The listing builds one solid part. Answer for the finished solid, in the listing's coordinates (mm). A direction names the side the tool comes from. Give positions to 0.01 mm unless a question says otherwise; leave off trailing zeros. Order: outer loops, then holes, each group sorted by start corner. A loop starts at its lowest first (then second) coordinate and runs counter-clockwise, first axis right, second up. Notation, with made-up numbers: (24, -25) - (75, -25) arc R18 cw to (75, -3) - close; hole circle Ø4 at (-20, 85). An arc over 180 degrees is marked (long way). Write each question's results on one line, items separated by ' | '. Start each with the question number.
1. Flat-ended cylindrical pins translate along their axes: pin 1 (2.5 mm diameter, centred on x = -33.5, z = -31.5, fed in from -Y); pin 2 (5 mm diameter, centred on y = -15.5, z = -8, fed in from -X); pin 3 (1 mm diameter, centred on x = -22, z = 27, fed in from -Y); pin 4 (0.8 mm diameter, centred on x = 5.5, z = -28.5, fed in from +Y). Find the tip coordinate at first contact, or state that the pin passes through.
2. Section A-A (z = -20) is taken. Give the vertices of the cut face in (x, y), and give its area (3 significant figures).
3. Determine the mould class of faces 5 (the face through (-2, -19, -28)), 6 (the face through (26, -29, -31)), 7 (the face through (27, 49, 0)) for opening direction Y: released by +Y, released by -Y, zero draft, split by the parting line, or undercut.
4. Section D-D (x = 26.5) is taken. Give the vertices of the cut face in (y, z) (3 decimals), and give its area (3 significant figures).
5. Find the intervals of material crossed by L1, parallel to X at y = -1.7, z = 24 (3 decimals); L2, parallel to X at y = -32.6, z = -31.5; L3, parallel to Z at x = -33.5, y = -32.1, in increasing order.
6. Section C-C (x = -6.5) is taken. Give the vertices of the cut face in (y, z).
7. Section B-B (y = 46.5) is taken. Give the vertices of the cut face in (x, z).
8. Which of the six approach directions +Z, -Z, +X, -X, +Y, -Y give full straight-line access (tool end or side, diameter ignored) to faces 1 (the face through (-33, -17, 31)), 2 (the face through (-2, -19, 28)), 3 (the face through (-36.929, -2.535, -25.013)), 4 (the face through (-13, -1, 29))?
from build123d import *

# Parameters (mm, degrees)
SKETCH1_W           = 58
SKETCH1_H           = 68
BOSS_EXTRUDE1_DEPTH = 4
SKETCH2_W           = 5
SKETCH2_H           = 68
BOSS_EXTRUDE2_DEPTH = 55
SKETCH3_W           = 70
SKETCH3_H           = 68
BOSS_EXTRUDE3_DEPTH = 5
CUT_EXTRUDE1_REACH  = 85.265
SKETCH4_R           = 1.375
CUT_EXTRUDE2_REACH  = 99.658
SKETCH5_R           = 1.375
SKETCH5_W           = 48
SKETCH5_H           = 35
CUT_EXTRUDE4_REACH  = 78.564
SKETCH6_W           = 46
SKETCH6_H           = 58
SKETCH7_W           = 62
SKETCH7_H           = 68
SKETCH7_W_2         = 50
SKETCH7_H_2         = 56
BOSS_EXTRUDE4_DEPTH = 24
SKETCH8_W           = 65
SKETCH8_H           = 68
SKETCH8_R           = 1.5
BOSS_EXTRUDE5_DEPTH = 5
SKETCH9_W           = 50
SKETCH9_H           = 56
CUT_EXTRUDE5_DEPTH  = 10
SKETCH10_W          = 58
SKETCH10_H          = 24
CUT_EXTRUDE6_DEPTH  = 10


with BuildPart() as part:
    # Sketch1 → Boss-Extrude1 (new body)
    with BuildSketch(Plane(origin=(0, 0, 0), x_dir=(1, 0, 0), z_dir=(0, 1, 0))):
        Rectangle(SKETCH1_W, SKETCH1_H)
    extrude(amount=BOSS_EXTRUDE1_DEPTH)

    # Sketch2 → Boss-Extrude2 (add)
    with BuildSketch(Plane(origin=(0, 4, 0), x_dir=(1, 0, 0), z_dir=(0, 1, 0))):
        with Locations((26.5, 0)):
            Rectangle(SKETCH2_W, SKETCH2_H)
    extrude(amount=BOSS_EXTRUDE2_DEPTH)

    # Sketch3 → Boss-Extrude3 (add)
    with BuildSketch(Plane.XZ):
        with Locations((-6, 0)):
            Rectangle(SKETCH3_W, SKETCH3_H)
    extrude(amount=BOSS_EXTRUDE3_DEPTH)

    # Sketch4 → Cut-Extrude1 (cut, up to next)
    with BuildSketch(Plane.XZ.offset(5), mode=Mode.PRIVATE) as cut_extrude1_sk1:
        with Locations(Location((-36, 24, 0), (0, 0, 270))):
            Circle(SKETCH4_R)
    cut_extrude1_tool1 = extrude(cut_extrude1_sk1.sketch, amount=-CUT_EXTRUDE1_REACH, mode=Mode.PRIVATE) & part.part
    # Sketch4 → Cut-Extrude1 (cut, up to next)
    with BuildSketch(Plane.XZ.offset(5), mode=Mode.PRIVATE) as cut_extrude1_sk2:
        with Locations(Location((-36, -24, 0), (0, 0, 90))):
            Circle(SKETCH4_R)
    cut_extrude1_tool2 = extrude(cut_extrude1_sk2.sketch, amount=-CUT_EXTRUDE1_REACH, mode=Mode.PRIVATE) & part.part
    add(cut_extrude1_tool1.solids().sort_by_distance((-36, -5, 24))[0], mode=Mode.SUBTRACT)
    add(cut_extrude1_tool2.solids().sort_by_distance((-36, -5, -24))[0], mode=Mode.SUBTRACT)

    # Sketch5 → Cut-Extrude2 (cut, up to next)
    with BuildSketch(Plane(origin=(29, 0, 0), x_dir=(0, 0, -1), z_dir=(1, 0, 0)), mode=Mode.PRIVATE) as cut_extrude2_sk1:
        with Locations((-31.5, 44)):
            Circle(SKETCH5_R)
    cut_extrude2_tool1 = extrude(cut_extrude2_sk1.sketch, amount=-CUT_EXTRUDE2_REACH, mode=Mode.PRIVATE) & part.part
    # Sketch5 → Cut-Extrude2 (cut, up to next)
    with BuildSketch(Plane(origin=(29, 0, 0), x_dir=(0, 0, -1), z_dir=(1, 0, 0)), mode=Mode.PRIVATE) as cut_extrude2_sk2:
        with Locations((-31.5, 11)):
            Circle(SKETCH5_R)
    cut_extrude2_tool2 = extrude(cut_extrude2_sk2.sketch, amount=-CUT_EXTRUDE2_REACH, mode=Mode.PRIVATE) & part.part
    # Sketch5 → Cut-Extrude2 (cut, up to next)
    with BuildSketch(Plane(origin=(29, 0, 0), x_dir=(0, 0, -1), z_dir=(1, 0, 0)), mode=Mode.PRIVATE) as cut_extrude2_sk3:
        with Locations((31.5, 11)):
            Circle(SKETCH5_R)
    cut_extrude2_tool3 = extrude(cut_extrude2_sk3.sketch, amount=-CUT_EXTRUDE2_REACH, mode=Mode.PRIVATE) & part.part
    # Sketch5 → Cut-Extrude2 (cut, up to next)
    with BuildSketch(Plane(origin=(29, 0, 0), x_dir=(0, 0, -1), z_dir=(1, 0, 0)), mode=Mode.PRIVATE) as cut_extrude2_sk4:
        with Locations((31.5, 44)):
            Circle(SKETCH5_R)
    cut_extrude2_tool4 = extrude(cut_extrude2_sk4.sketch, amount=-CUT_EXTRUDE2_REACH, mode=Mode.PRIVATE) & part.part
    # Sketch5 → Cut-Extrude2 (cut, up to next)
    with BuildSketch(Plane(origin=(29, 0, 0), x_dir=(0, 0, -1), z_dir=(1, 0, 0)), mode=Mode.PRIVATE) as cut_extrude2_sk5:
        with Locations((0, 31.5)):
            Rectangle(SKETCH5_W, SKETCH5_H)
    cut_extrude2_tool5 = extrude(cut_extrude2_sk5.sketch, amount=-CUT_EXTRUDE2_REACH, mode=Mode.PRIVATE) & part.part
    add(cut_extrude2_tool1.solids().sort_by_distance((29, 44, 31.5))[0], mode=Mode.SUBTRACT)
    add(cut_extrude2_tool2.solids().sort_by_distance((29, 11, 31.5))[0], mode=Mode.SUBTRACT)
    add(cut_extrude2_tool3.solids().sort_by_distance((29, 11, -31.5))[0], mode=Mode.SUBTRACT)
    add(cut_extrude2_tool4.solids().sort_by_distance((29, 44, -31.5))[0], mode=Mode.SUBTRACT)
    add(cut_extrude2_tool5.solids().sort_by_distance((29, 31.5, 0))[0], mode=Mode.SUBTRACT)

    # Sketch6 → Cut-Extrude4 (cut, up to next)
    with BuildSketch(Plane(origin=(0, 4, 0), x_dir=(1, 0, 0), z_dir=(0, 1, 0)), mode=Mode.PRIVATE) as cut_extrude4_sk1:
        with Locations((-4, 0)):
            Rectangle(SKETCH6_W, SKETCH6_H)
    cut_extrude4_tool1 = extrude(cut_extrude4_sk1.sketch, amount=-CUT_EXTRUDE4_REACH, mode=Mode.PRIVATE) & part.part
    add(cut_extrude4_tool1.solids().sort_by_distance((-4, 4, 0))[0], mode=Mode.SUBTRACT)

    # Sketch7 → Boss-Extrude4 (add)
    with BuildSketch(Plane.XZ.offset(5)):
        with Locations((-2, 0)):
            Rectangle(SKETCH7_W, SKETCH7_H)
        with Locations((-2, 0)):
            Rectangle(SKETCH7_W_2, SKETCH7_H_2, mode=Mode.SUBTRACT)
    extrude(amount=BOSS_EXTRUDE4_DEPTH)

    # Sketch8 → Boss-Extrude5 (add)
    with BuildSketch(Plane.XZ.offset(29)):
        with Locations((-3.5, 0)):
            Rectangle(SKETCH8_W, SKETCH8_H)
        with Locations(Location((26.5, -31.5, 0), (0, 0, 270))):
            Circle(SKETCH8_R, mode=Mode.SUBTRACT)
        with Locations(Location((-33.5, -31.5, 0), (0, 0, 70.528779366))):
            Circle(SKETCH8_R, mode=Mode.SUBTRACT)
        with Locations(Location((-33.5, 31.5, 0), (0, 0, 70.528779366))):
            Circle(SKETCH8_R, mode=Mode.SUBTRACT)
        with Locations(Location((26.5, 31.5, 0), (0, 0, 270))):
            Circle(SKETCH8_R, mode=Mode.SUBTRACT)
        with Locations(Location((-3.5, 0, 0), (0, 0, 270))):
            Circle(SKETCH8_R, mode=Mode.SUBTRACT)
    extrude(amount=BOSS_EXTRUDE5_DEPTH)

    # Sketch9 → Cut-Extrude5 (cut)
    with BuildSketch(Plane(origin=(0, -29, 0), x_dir=(1, 0, 0), z_dir=(0, 1, 0))):
        with Locations((-2, 0)):
            Rectangle(SKETCH9_W, SKETCH9_H)
    extrude(amount=-CUT_EXTRUDE5_DEPTH, mode=Mode.SUBTRACT)

    # Sketch10 → Cut-Extrude6 (cut)
    with BuildSketch(Plane.ZY.offset(33)):
        with Locations((0, -17)):
            Rectangle(SKETCH10_W, SKETCH10_H)
    extrude(amount=-CUT_EXTRUDE6_DEPTH, mode=Mode.SUBTRACT)


solid = part.part
Reported:
1) pin 1: y = -29 | pin 2: x = 23 | pin 3: through | pin 4: y = -5
2) outline: (-41, -5) - (-27, -5) - (-27, 4) - (-29, 4) - (-29, 0) - (-41, 0) - close; (-36, -34) - (-27, -34) - (-27, -29) - (-36, -29) - close; (19, -5) - (23, -5) - (23, -34) - (29, -34) - (29, 14) - (24, 14) - (24, 4) - (19, 4) - close; (24, 49) - (29, 49) - (29, 59) - (24, 59) - close | area: 487 mm²
3) face 5: zero draft | face 6: released by -Y | face 7: undercut
4) outline: (-34, -34) - (59, -34) - (59, 34) - (-34, 34) - (-34, 33) - (-29, 33) - (-29, 30) - (-34, 30) - (-34, -30) - (-29, -30) - (-29, -33) - (-34, -33) - close; hole circle Ø2.75 at (11, -31.5); hole circle Ø2.75 at (11, 31.5); hole (14, -24) - (49, -24) - (49, 24) - (14, 24) - close; hole circle Ø2.75 at (44, -31.5); hole circle Ø2.75 at (44, 31.5) | area: 4,590 mm²
5) L1: -41 to -37.375, -34.625 to -27, 19 to 29 | L2: -36 to -35, -32 to 25, 28 to 29 | L3: -34 to -33, -30 to 30, 33 to 34
6) outline: (-34, -34) - (4, -34) - (4, -29) - (-5, -29) - (-5, -28) - (-34, -28) - close; (-34, 28) - (-5, 28) - (-5, 29) - (4, 29) - (4, 34) - (-34, 34) - close
7) outline: (24, -34) - (29, -34) - (29, -24) - (24, -24) - close; (24, 24) - (29, 24) - (29, 34) - (24, 34) - close
8) face 1: +Z, -Z, -X | face 2: -Y | face 3: +Y | face 4: none
